The drawing under review shows one solid part. Ordinate dimensions are in mm from its lowest x, y, z. Coordinates: 2 decimals unless noted, no trailing zeros. Order: outer loops, then holes, each group sorted by start corner. A loop starts at its lowest first (then second) coordinate and runs counter-clockwise, first axis right, second up.
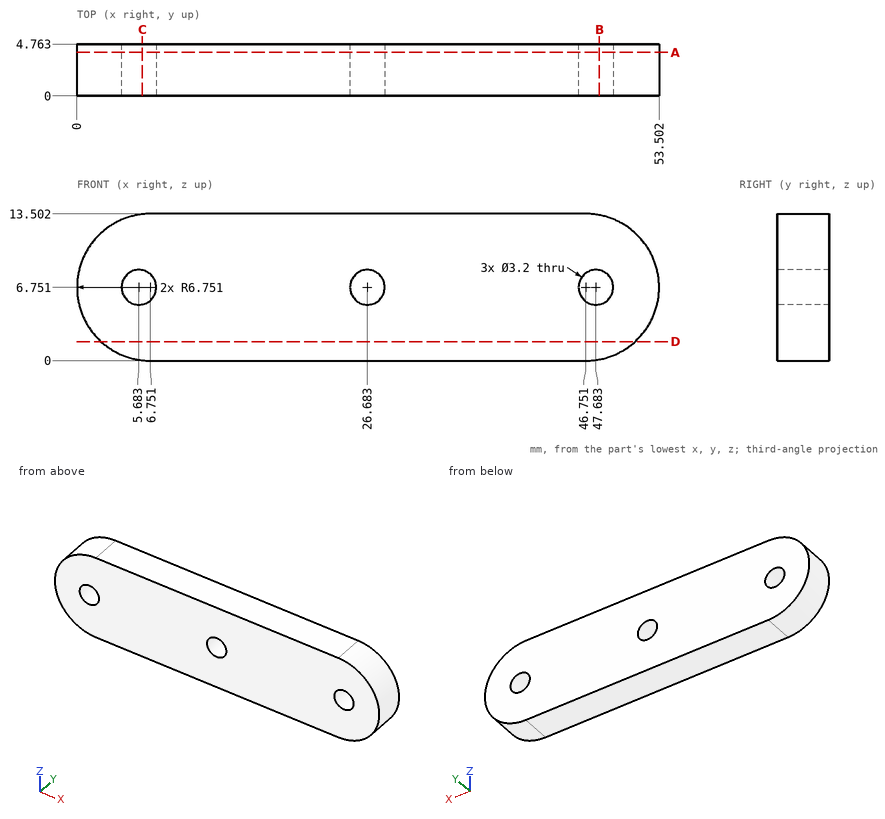
(1) Wall thickness on probe 1 along X at (y, z) = (2.9, 8) (1 decimal); probe 2 along X at (y, z) = (3.8, 6.25); probe 3 along Z at (x, y) = (7, 1.15): over which ranges is each line inside the solid? List them lowest first.
A:
probe 1: x = 0.1 to 4.7, 6.7 to 25.7, 27.7 to 46.7, 48.7 to 53.4
probe 2: x = 0.02 to 4.16, 7.2 to 25.16, 28.2 to 46.16, 49.2 to 53.48
probe 3: z = 0 to 5.84, 7.66 to 13.5
(2) We need section D-D, the plane z = 1.75. Write out the cut boundary in (x, y), and give its area (3 significant figures).
A:
outline: (2.22, 0) - (51.29, 0) - (51.29, 4.76) - (2.22, 4.76) - close
area: 234 mm2
(3) We need section A-A, the plane y = 4. Write out the cut boundary in (x, z).
A:
outline: (6.75, 0) - (46.75, 0) arc R6.75 ccw to (46.75, 13.5) - (6.75, 13.5) arc R6.75 ccw to start; hole circle Ø3.2 at (5.68, 6.75); hole circle Ø3.2 at (26.68, 6.75); hole circle Ø3.2 at (47.68, 6.75)
(4) We need section C-C, the plane x = 6. Write out the cut boundary in (y, z), and give its area (3 significant figures).
A:
outline: (0, 0.04) - (4.76, 0.04) - (4.76, 5.18) - (0, 5.18) - close; (0, 8.32) - (4.76, 8.32) - (4.76, 13.46) - (0, 13.46) - close
area: 49.0 mm2
(5) We need section B-B, the plane x = 48. Write out the cut boundary in (y, z) (1 decimal).
A:
outline: (0, 0.1) - (4.8, 0.1) - (4.8, 5.2) - (0, 5.2) - close; (0, 8.3) - (4.8, 8.3) - (4.8, 13.4) - (0, 13.4) - close
